Autodesk Inventor part; units mm, degrees
ref_plane "YZ Plane" through (0, 0, 0) normal (1, 0, 0) x (0, 1, 0)
ref_plane "XZ Plane" through (0, 0, 0) normal (0, 1, 0) x (-1, 0, 0)
ref_plane "XY Plane" through (0, 0, 0) normal (0, 0, 1) x (1, 0, 0)
sketch "Sketch1" plane through (0, 0, 0) normal (1, 0, 0) x (0, 1, 0)
  circle A0 centre (0, 0) radius 12.7
  circle A1 centre (0, 0) radius 1.5875
  line L0 (-12.7, 0) -> (-1.5875, 0)
  circle A2 centre (-7.62, 0) radius 1.5875
  dimension "d0" = 25.4
  dimension "d1" = 3.175
  dimension "d2" = 3.175
  dimension "d3" = 5.08
extrude "Extrusion1" add sketch "Sketch1" along normal blind 3.175
properties part number "CURM_Caterpillar_wheel"
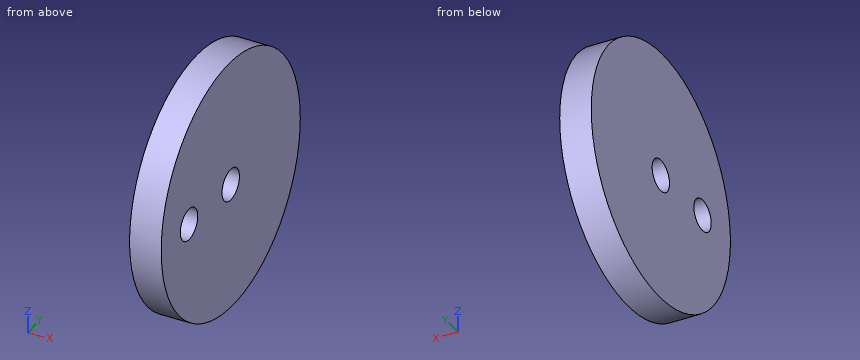
Input: part model. Units: mm. Frame: model coordinates. Give positions to 0.01 mm unless a question says otherwise; leave off trailing zeros. Order: outer loops, then holes, each group sorted by start corner. A loop starts at its lowest first (then second) coordinate and runs counter-clockwise, first axis right, second up. Notation, with made-up numbers: M -22.5,81.25 L 12.5,81.25 A12 cw 12.5,98.25 Z; hole C 26.25,77.5 d2. An arc over 180 degrees is marked long. One line per question, with ' | ' between items.
1) Ray query, L1, parallel to Y at x = 2.1, z = 0; L2, parallel to Z at x = 1.25, y = 0; L3, parallel to Z at x = 0.7, y = -7.75. Return the intervals inside material, ascending.
Filled in:
L1: y = -12.7 to -9.21, -6.03 to -1.59, 1.59 to 12.7 | L2: z = -12.7 to -1.59, 1.59 to 12.7 | L3: z = -10.06 to -1.58, 1.58 to 10.06
2) Section C-C on x = 1.1. Output: boundary loops of the cut face in (y, z) (1 decimal).
Filled in:
outline: C 0,0 d25.4; hole C -7.6,0 d3.2; hole C 0,0 d3.2
3) Section B-B on y = 0. Output: boundary loops of the cut face in (x, z) (1 decimal).
Filled in:
outline: M 0,-12.7 L 3.2,-12.7 L 3.2,-1.6 L 0,-1.6 Z; M 0,1.6 L 3.2,1.6 L 3.2,12.7 L 0,12.7 Z
4) Section D-D on y = -7.62. Output: boundary loops of the cut face in (x, z) (1 decimal), and give its area (3 significant figures).
Filled in:
outline: M 0,-10.2 L 3.2,-10.2 L 3.2,-1.6 L 0,-1.6 Z; M 0,1.6 L 3.2,1.6 L 3.2,10.2 L 0,10.2 Z | area: 54.4 mm2
5) Section A-A on z = 0. Output: boundary loops of the cut face in (x, y) (1 decimal), and give its area (3 significant figures).
Filled in:
outline: M 0,-12.7 L 3.2,-12.7 L 3.2,-9.2 L 0,-9.2 Z; M 0,-6 L 3.2,-6 L 3.2,-1.6 L 0,-1.6 Z; M 0,1.6 L 3.2,1.6 L 3.2,12.7 L 0,12.7 Z | area: 60.5 mm2
6) Contact query for flat-ended pins moving along their axis: P1, Ø1.9, axis at y = 0, z = 0, coming from the -X side; P2, Ø1, axis at x = 3, z = -2.5, coming from the +Y side. Output: stop coordinate, or through.
Filled in:
P1: passes through | P2: stops at y = 12.54
